Input: part model. Units: mm. Frame: model coordinates. A direction names the side the tool comes from. Give positions to 0.01 mm unless a question says otherwise; leave off trailing zeros. Loops run counter-clockwise (first coordinate to the right, second up) from the corner with the lowest first, then second, coordinate; pieces in that order, holes last.
from build123d import *

# Parameters (mm, degrees)
CYLINDER004_R     = 1.6
CYLINDER004_DEPTH = 7
BOX008_W          = 11
BOX008_H          = 3.4
BOX008_DEPTH      = 8.4
CYLINDER003_R     = 1.6
CYLINDER003_DEPTH = 7
BOX007_W          = 3
BOX007_H          = 10
BOX007_DEPTH      = 6
FILLET003_R       = 3
BOX009_W          = 9
BOX009_H          = 2
BOX009_DEPTH      = 23.4
BOX006_W          = 3
BOX006_H          = 51
BOX006_DEPTH      = 29
FILLET002_R       = 10


with BuildPart() as screw_hole_cylinder003:
    # Cylinder004 → Cylinder004 (new body)
    with BuildSketch(Plane(origin=(-6, 15, 10), x_dir=(0, 0, -1), z_dir=(1, 0, 0))):
        Circle(CYLINDER004_R)
    extrude(amount=CYLINDER004_DEPTH)


with BuildPart() as wire_extract_cube001:
    # Box008 → Box008 (new body)
    with BuildSketch(Plane(origin=(-4, 22, -4.2), x_dir=(1, 0, 0), z_dir=(0, 0, 1))):
        with Locations((5.5, 1.7)):
            Rectangle(BOX008_W, BOX008_H)
    extrude(amount=BOX008_DEPTH)


with BuildPart() as cover_extract_fusion:
    # Part__Mirroring004: instance of screw hole cylinder003
    add(screw_hole_cylinder003.part.mirror(Plane(origin=(0, 0, 0), x_dir=(0, 1, 0), z_dir=(0, 0, 1))))

    # Fusion002: union screw hole cylinder003, wire extract cube001
    add(screw_hole_cylinder003.part)
    add(wire_extract_cube001.part)


with BuildPart() as screw_hole_cylinder002:
    # Cylinder003 → Cylinder003 (new body)
    with BuildSketch(Plane(origin=(-7, -18, 16), x_dir=(0, 0, -1), z_dir=(1, 0, 0))):
        Circle(CYLINDER003_R)
    extrude(amount=CYLINDER003_DEPTH)


with BuildPart() as cut002:
    # Box007 → Box007 (new body)
    with BuildSketch(Plane(origin=(-4, -23, 13), x_dir=(1, 0, 0), z_dir=(0, 0, 1))):
        with Locations((1.5, 5)):
            Rectangle(BOX007_W, BOX007_H)
    extrude(amount=BOX007_DEPTH)

    # Fillet003
    fillet003_edges = [cut002.edges().sort_by_distance(p)[0] for p in [
        (-2.5, -23, 19),
        (-2.5, -13, 19),
    ]]
    fillet(fillet003_edges, radius=FILLET003_R)

    # Cut002: cut screw hole cylinder002
    add(screw_hole_cylinder002.part, mode=Mode.SUBTRACT)


with BuildPart() as part_mirroring003:
    # Part__Mirroring003: instance of Cut002
    add(cut002.part.mirror(Plane(origin=(0, 0, 0), x_dir=(0, 1, 0), z_dir=(0, 0, 1))))


with BuildPart() as external_cube_border:
    # Box009 → Box009 (new body)
    with BuildSketch(Plane(origin=(-10.6, -23, -11.7), x_dir=(1, 0, 0), z_dir=(0, 0, 1))):
        with Locations((4.5, 1)):
            Rectangle(BOX009_W, BOX009_H)
    extrude(amount=BOX009_DEPTH)


with BuildPart() as cover_cut:
    # Box006 → Box006 (new body)
    with BuildSketch(Plane(origin=(-4, -23, -14.5), x_dir=(1, 0, 0), z_dir=(0, 0, 1))):
        with Locations((1.5, 25.5)):
            Rectangle(BOX006_W, BOX006_H)
    extrude(amount=BOX006_DEPTH)

    # Fillet002
    fillet002_edges = [cover_cut.edges().sort_by_distance(p)[0] for p in [
        (-2.5, 28, -14.5),
        (-2.5, 28, 14.5),
    ]]
    fillet(fillet002_edges, radius=FILLET002_R)

    # Fusion003: union Part__Mirroring003, Cut002, external cube border
    add(part_mirroring003.part)
    add(cut002.part)
    add(external_cube_border.part)

    # Cut003: cut cover extract fusion
    add(cover_extract_fusion.part, mode=Mode.SUBTRACT)


solid = cover_cut.part
(1) Cut plane C-C (z = -3). Return the cut outline in (x, y), and give its area (3 significant figures).
Values follow:
outline: (-10.6, -23) - (-1, -23) - (-1, 22) - (-4, 22) - (-4, -21) - (-10.6, -21) - close; (-4, 25.4) - (-1, 25.4) - (-1, 28) - (-4, 28) - close
area: 156 mm2
(2) Reachability of faces 1 (the flat face through (-7, -22, -11.7)), 2 (the flat face through (-10.6, -22, 0)), 3 (the flat face through (-3, 28, 0)), 4 (the flat face through (-3, 24, -4.2)), 5 (the flat face through (-3, -13, 15)) from +Z, -Z, +X, -X, +Y, -Y: full face, straight path, thin tool, end or side. Return the list, or none.
Values follow:
face 1: -Z, -X, +Y, -Y
face 2: +Z, -Z, -X, +Y, -Y
face 3: +Z, -Z, +X, -X, +Y
face 4: +X, -X
face 5: +Z, +X, -X, +Y
(3) Cut plane A-A (y = -18). Return the cut outline in (x, z).
Values follow:
outline: (-4, -19) - (-1, -19) - (-1, -17.6) - (-4, -17.6) - close; (-4, -14.5) - (-1, -14.5) - (-1, 14.5) - (-4, 14.5) - close; (-4, 17.6) - (-1, 17.6) - (-1, 19) - (-4, 19) - close
(4) Pin query (flat end, axial travel): pin 1 Ø8 at (y, z) = (14, -5.5) entering from -X; pin 2 Ø1.6 at (x, y) = (-6, -22) entering from -Z; pin 3 Ø2 at (x, z) = (-5.5, -11.5) entering from +Y; pin 4 Ø4 at (y, z) = (15, 10) entering from +X. Return the tip coordinate at first contact, or that it passes through.
Values follow:
pin 1: stops at x = -4
pin 2: stops at z = -11.7
pin 3: stops at y = -21
pin 4: stops at x = -1
(5) Cut plane B-B (x = -3.25). Return the cut outline in (y, z), and give its area (3 significant figures).
Values follow:
outline: (-23, -16) arc R3 ccw to (-20, -19) - (-16, -19) arc R3 ccw to (-13, -16) - (-13, -14.5) - (18, -14.5) arc R10 ccw to (28, -4.5) - (28, 4.5) arc R10 ccw to (18, 14.5) - (-13, 14.5) - (-13, 16) arc R3 ccw to (-16, 19) - (-20, 19) arc R3 ccw to (-23, 16) - close; hole (-18.56, -14.5) arc R1.6 ccw (long way) to (-17.44, -14.5) - close; hole (-18.56, 14.5) - (-17.44, 14.5) arc R1.6 ccw (long way) to start; hole circle Ø3.2 at (15, -10); hole circle Ø3.2 at (15, 10); hole (22, -4.2) - (25.4, -4.2) - (25.4, 4.2) - (22, 4.2) - close
area: 1,460 mm2
(6) Mould query, pull axis Z, two halves, no side actions, for faces 6 (the cylindrical face through (-2.52, -17.94, -17.6)), 7 (the flat face through (-7, -22, 11.7)), 8 (the flat face through (-6, -23, 0)). Classes: +Z half, -Z half, draft (parallel to the pull), parting line (faces both ways), or undercut.
Values follow:
face 6: undercut
face 7: +Z half
face 8: draft
(7) Cut plane D-D (z = -11). Return the cut outline in (x, y), and give its area (3 significant figures).
Values follow:
outline: (-10.6, -23) - (-1, -23) - (-1, 13.75) - (-4, 13.75) - (-4, -21) - (-10.6, -21) - close; (-4, 16.25) - (-1, 16.25) - (-1, 25.6) - (-4, 25.6) - close
area: 152 mm2
(8) Ray query, probe 1 along Z at (x, y) = (-2.6, -18); probe 2 along Y at (x, z) = (-2.25, 16); probe 3 along X at (y, z) = (-11.5, 12.5). Return the intervals inside material, ascending.
Values follow:
probe 1: z = -19 to -17.6, -14.5 to 14.5, 17.6 to 19
probe 2: y = -23 to -19.6, -16.4 to -13
probe 3: x = -4 to -1
